from build123d import *

# Parameters (mm, degrees)
SKETCH1_W           = 192.921126566
SKETCH1_H           = 64.543351392
SKETCH1_W_2         = 152.4
SKETCH1_H_2         = 25.4
BOSS_EXTRUDE4_DEPTH = 50.8
CHAMFER2_SIZE       = 38.1
SKETCH1_5_W         = 152.4
SKETCH1_5_H         = 25.4
CUT_EXTRUDE1_DEPTH  = 35.56


with BuildPart() as part:
    # Sketch1 → Boss-Extrude4 (new body)
    # profile 1 of 2: a face of its own
    with BuildSketch(Plane(origin=(0, 0, 0), x_dir=(1, 0, 0), z_dir=(0, 1, 0))):
        Rectangle(SKETCH1_W, SKETCH1_H)
        Rectangle(SKETCH1_W_2, SKETCH1_H_2, mode=Mode.SUBTRACT)
    # profile 2 of 2: a face of its own
    with BuildSketch(Plane(origin=(0, 0, 0), x_dir=(1, 0, 0), z_dir=(0, 1, 0))):
        Rectangle(SKETCH1_W_2, SKETCH1_H_2)
    extrude(amount=-BOSS_EXTRUDE4_DEPTH)

    # Chamfer2
    # the kernel refuses this chamfer: 38.1 mm, written as the material it takes off along each edge
    with BuildSketch(Plane(origin=(-194.441685124, -50.8, 32.271675696), x_dir=(0, 0.9996219169112968, 0.02749587661058638), z_dir=(1, 0, 0))) as chamfer2_piece_1:
        Polygon((CHAMFER2_SIZE * 0.999621916911, -CHAMFER2_SIZE * 0.0274958766106), (-CHAMFER2_SIZE * 0.0274958766106, -CHAMFER2_SIZE * 0.999621916911), (0, 0), align=None)
    extrude(amount=388.883370249, mode=Mode.SUBTRACT)
    with BuildSketch(Plane(origin=(194.441685124, -50.8, -32.271675696), x_dir=(0, -0.02749587661058638, 0.9996219169112968), z_dir=(-1, 0, 0))) as chamfer2_piece_2:
        Polygon((CHAMFER2_SIZE * 0.999621916911, CHAMFER2_SIZE * 0.0274958766106), (-CHAMFER2_SIZE * 0.0274958766106, CHAMFER2_SIZE * 0.999621916911), (0, 0), align=None)
    extrude(amount=388.883370249, mode=Mode.SUBTRACT)

    # Sketch1<5> → Cut-Extrude1 (cut)
    with BuildSketch(Plane(origin=(0, 0, 0), x_dir=(1, 0, 0), z_dir=(0, 1, 0))):
        Rectangle(SKETCH1_5_W, SKETCH1_5_H)
    extrude(amount=-CUT_EXTRUDE1_DEPTH, mode=Mode.SUBTRACT)


solid = part.part
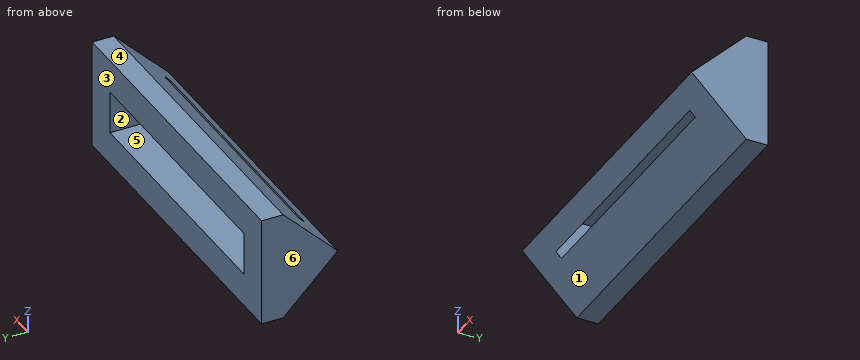
Source: CAD feature listing. Evaluate the final solid. Frame: model axes, mm. Face numbers are marked on the shaded views. A direction names the side the tool comes from. Round coordinates to 2 decimals unless told otherwise and drop trailing zeros. Order: outer loops, then holes, each group sorted by start corner. A loop starts at its lowest first (then second) coordinate and runs counter-clockwise, first axis right, second up. Notation, with made-up numbers: (89.25, 87.25) - (148.25, 87.25) arc R21 ccw to (148.25, 122.25) - close; hole circle Ø9 at (10, 31). An arc over 180 degrees is marked (long way). Use a Markdown table: item, result. Add a question column.
1. Mould query, pull axis Z, two halves, no side actions, for the marked faces 1, 2, 3 and 4. Classes: +Z half, -Z half, draft (parallel to the pull), parting line (faces both ways), or undercut.
2. Set-up query: the marked faces 5 and 6. Return all of +Z, -Z, +X, -X, +Y, -Y with unobstructed straight access to the full face (end or side cutting, diameter ignored); none if empty.
3. Section query B-B (y = -10). Return the cut outline in (x, z).
4. Section query D-D (y = -29). Return the cut outline in (x, z).
5. First-contact query: pin 1 (1 mm diameter, centred on x = 32, y = -24, fed in from +Z); pin 2 (1.5 mm diameter, centred on x = -31, y = -30.5, fed in from +Z); pin 3 (4 mm diameter, centred on x = -50.5, y = -24, fed in from +Z). Flat tips, straight axial feed; report the tip coordinate or a pass-through.
6. Line query: probe 1 along X at (y, z) = (-13, -11.5); probe 2 along Z at (x, y) = (-18, -4.5); probe 3 along Z at (x, y) = (30, -22). Output: solid intervals per line, ascending.
7. Section query A-A (x = -37.5). Return the cut outline in (y, z), then the cut area to 3 significant figures.
8. Section query C-C (z = 28.5). Return the cut outline in (x, y).
Derived:
| question | item | result |
|---|---|---|
| 1 | face 1 | -Z half |
| 1 | face 2 | undercut |
| 1 | face 3 | draft |
| 1 | face 4 | +Z half |
| 2 | face 5 | +Y, -Y |
| 2 | face 6 | +Z, -Z, -X, +Y, -Y |
| 3 | outline | (-96.46, -32.27) - (96.46, -32.27) - (96.46, 32.27) - (-96.46, 32.27) - close; hole (-76.2, -12.7) - (76.2, -12.7) - (76.2, 12.7) - (-76.2, 12.7) - close |
| 4 | outline | (-96.46, -15.97) - (96.46, -15.97) - (96.46, 15.97) - (-96.46, 15.97) - close; hole (-76.2, -12.7) - (76.2, -12.7) - (76.2, 12.7) - (-76.2, 12.7) - close |
| 5 | pin 1 | z = 21.47 |
| 5 | pin 2 | z = 15.22 |
| 5 | pin 3 | z = 22.97 |
| 6 | probe 1 | -96.46 to -76.2, 76.2 to 96.46 |
| 6 | probe 2 | -32.27 to -12.7, 12.7 to 32.27 |
| 6 | probe 3 | -22.97 to -12.7, 12.7 to 22.97 |
| 7 | outline | (-44.97, 0) - (-35.56, -9.41) - (-35.56, 9.41) - close; (-32.27, -12.7) - (-12.7, -32.27) - (0, -32.27) - (0, -12.7) - close; (-32.27, 12.7) - (0, 12.7) - (0, 32.27) - (-12.7, 32.27) - close |
| 7 | area | 969 mm2 |
| 8 | outline | (-96.46, -16.47) - (96.46, -16.47) - (96.46, 0) - (-96.46, 0) - close |
